The model under review builds one solid part; all positions refer to its coordinate system, in mm. A direction names the side the tool comes from. Round coordinates to 2 decimals unless told otherwise and drop trailing zeros. Order: outer loops, then holes, each group sorted by start corner. A loop starts at its lowest first (then second) coordinate and runs counter-clockwise, first axis right, second up. Notation, with made-up numbers: M -7.75,31.5 L 31.25,31.5 A21 ccw 31.25,52.5 Z; hole C 8,47.5 d1. An arc over 180 degrees is marked long. Use a Markdown table: item, result. Add a question column.
1. The part is to be moulded in two halves that separate along Z. For faces 1 (the cylindrical face through (1.521, 52.752, 5.599)), 2 (the cylindrical face through (3.9, 1.52, 45.14)), 3 (the flat face through (19, 0, 23)), say which applies: +Z half, -Z half, draft (parallel to the pull), parting line (faces both ways), or undercut.
2. For faces 4 (the flat face through (1, 51, 31)), 5 (the flat face through (37, 2, 23)), 6 (the flat face through (3, 36, 16)), list the 3-axis set-ups (+Z, -Z, +X, -X, +Y, -Y) from which the entire face can be reached by the end or side of a thin tool; tool diameter is ignored.
3. Consider section C-C on z = 20.5. State the section outline as (x, y) points, then the cut area to 3 significant figures.
4. Consider section D-D on y = 13.5. State the section outline as (x, z) points, then the cut area to 3 significant figures.
5. Insertion check: P1, Ø1, axis at y = 12.5, z = 30.5, coming from the -X side; P2, Ø6, axis at x = 21.5, z = 34.5, coming from the +Y side; P3, Ø3.5, axis at x = 1.5, y = 46.5, coming from the +Z side; P4, Ø5, axis at x = 2, y = 13, coming from the +Z side. Each pin has a flat end and moves straight along its axis. Give the tip position at first contact, or say it passes through.
6. Consider section B-B on y = 55. State the section outline as (x, z) points.
7. Consider section A-A on z = 25.5. State the section outline as (x, y) points, then the cut area to 3 significant figures.
8. To check wall thickness, follow probe 1 along Z at (x, y) = (1.7, 55); probe 2 along Y at (x, z) = (22.5, 42). State the ranges of each line that lie inside material, in increasing order.
from build123d import *

# Parameters (mm, degrees)
BOSS_EXTRUDE1_DEPTH = 46
CUT_EXTRUDE1_DEPTH  = 3
SKETCH3_R           = 2.25
CUT_EXTRUDE2_DEPTH  = 46
FILLET1_R           = 3


with BuildPart() as part:
    # Sketch1 → Boss-Extrude1 (new body)
    with BuildSketch(Plane.XY):
        Polygon((0, 0), (0, 65), (3, 65), (3, 3), (37, 3), (37, 0), align=None)
    extrude(amount=BOSS_EXTRUDE1_DEPTH)

    # Sketch2 → Cut-Extrude1 (cut)
    with BuildSketch(Plane.ZY):
        Polygon((32, 65), (46, 65), (46, 0), (32, 0), (32, 40), (31, 40), (31, 65), align=None)
    extrude(amount=-CUT_EXTRUDE1_DEPTH, mode=Mode.SUBTRACT)

    # Sketch3 → Cut-Extrude2 (cut)
    with BuildSketch(Plane(origin=(3, 0, 0), x_dir=(0, 0, -1), z_dir=(1, 0, 0))):
        with Locations(Location((-25.5, 55, 0), (0, 0, 90))):
            Circle(SKETCH3_R)
        with Locations(Location((-5.5, 55, 0), (0, 0, 90))):
            Circle(SKETCH3_R)
    extrude(amount=-CUT_EXTRUDE2_DEPTH, mode=Mode.SUBTRACT)

    # Fillet1
    # the kernel refuses this fillet: 3 mm, written as the material it adds along each edge
    with BuildSketch(Plane(origin=(3, 3, 0), x_dir=(0, 1, 0), z_dir=(0, 0, 1))) as fillet1_piece_1:
        with BuildLine():
            CenterArc((FILLET1_R, -FILLET1_R), FILLET1_R, 90, 90)
            Line((0, -FILLET1_R), (0, 0))
            Line((0, 0), (FILLET1_R, 0))
        make_face()
    extrude(amount=32)
    # the kernel refuses this fillet: 3 mm, written as the material it takes off along each edge
    with BuildSketch(Plane(origin=(37, 10.5, 46), x_dir=(0, 0, -1), z_dir=(0, -1, 0)), Plane(origin=(37, 10.5, 0), x_dir=(-1, 0, 0), z_dir=(0, -1, 0)), Plane(origin=(-7.5, 65, 0), x_dir=(0, -1, 0), z_dir=(1, 0, 0)), Plane(origin=(-7.5, 65, 31), x_dir=(0, 0, -1), z_dir=(1, 0, 0))) as fillet1_2_piece_1:
        with BuildLine():
            CenterArc((FILLET1_R, -FILLET1_R), FILLET1_R, 90, 90)
            Line((0, -FILLET1_R), (0, 0))
            Line((0, 0), (FILLET1_R, 0))
        make_face()
    extrude(amount=18, mode=Mode.SUBTRACT)
    with BuildSketch(Plane(origin=(3, 10.5, 46), x_dir=(0, 0, -1), z_dir=(0, -1, 0))) as fillet1_2_piece_2:
        with BuildLine():
            CenterArc((FILLET1_R, FILLET1_R), FILLET1_R, 180, 90)
            Line((0, FILLET1_R), (0, 0))
            Line((0, 0), (FILLET1_R, 0))
        make_face()
    extrude(amount=18, mode=Mode.SUBTRACT)
    with BuildSketch(Plane(origin=(-5.590169944, 40, 32), x_dir=(0, -1, 0), z_dir=(1, 0, 0))) as fillet1_2_piece_3:
        with BuildLine():
            CenterArc((2.236067977, 3), FILLET1_R, 221.810314896, 48.189685104)
            Line((0, 1), (0, 0))
            Line((0, 0), (2.236067977, 0))
        make_face()
    extrude(amount=14.180339887, mode=Mode.SUBTRACT)


solid = part.part
Answer block:
| question | item | result |
|---|---|---|
| 1 | face 1 | undercut |
| 1 | face 2 | +Z half |
| 1 | face 3 | draft |
| 2 | face 4 | +Z, +X, -X, +Y |
| 2 | face 5 | +Z, -Z, +X, +Y, -Y |
| 2 | face 6 | +Z, -Z, +X, +Y |
| 3 | outline | M 0,0 L 37,0 L 37,3 L 6,3 A3 cw 3,6 L 3,65 L 0,65 Z |
| 3 | area | 299 mm^2 |
| 4 | outline | M 0,0 L 3,0 L 3,32 L 0,32 Z |
| 4 | area | 96.0 mm^2 |
| 5 | P1 | x = 0 |
| 5 | P2 | y = 3 |
| 5 | P3 | z = 31 |
| 5 | P4 | z = 32 |
| 6 | outline | M 0,0 L 3,0 L 3,3.25 L 0,3.25 Z; M 0,7.75 L 3,7.75 L 3,23.25 L 0,23.25 Z; M 0,27.75 L 3,27.75 L 3,31 L 0,31 Z |
| 7 | outline | M 0,0 L 37,0 L 37,3 L 6,3 A3 cw 3,6 L 3,52.75 L 0,52.75 Z; M 0,57.25 L 3,57.25 L 3,65 L 0,65 Z |
| 7 | area | 285 mm^2 |
| 8 | probe 1 | 0 to 3.25, 7.75 to 23.25, 27.75 to 31 |
| 8 | probe 2 | 0 to 3 |
